```python
from build123d import *

# Parameters (mm, degrees)
ESQUISSE1_W              = 148
ESQUISSE1_H              = 330
BOSS_EXTRU_1_DEPTH       = 6
ESQUISSE2_W              = 30
ESQUISSE2_H              = 6
ESQUISSE2_W_2            = 6
ESQUISSE2_H_2            = 40
ENL_V_MAT_EXTRU_1_DEPTH  = 6
ESQUISSE6_W              = 6
ESQUISSE6_H              = 60
ENL_V_MAT_EXTRU_4_DEPTH  = 10
ESQUISSE8_W              = 6
ESQUISSE8_H              = 330
BOSS_EXTRU_2_DEPTH       = 57
ENL_V_MAT_EXTRU_5_DEPTH  = 389.536999525
ESQUISSE10_W             = 30
ESQUISSE10_H             = 6
ENL_V_MAT_EXTRU_6_DEPTH  = 389.536999525
ENL_V_MAT_EXTRU_9_DEPTH  = 389.536999525
ENL_V_MAT_EXTRU_11_DEPTH = 10
ESQUISSE16_R             = 1.5
ENL_V_MAT_EXTRU_12_DEPTH = 6
ESQUISSE17_R             = 2.995
ENL_V_MAT_EXTRU_13_DEPTH = 3
ESQUISSE18_R             = 9
ESQUISSE18_W             = 28.5
ESQUISSE18_H             = 12.5
ENL_V_MAT_EXTRU_14_DEPTH = 389.536999525
ESQUISSE5_W              = 30
ESQUISSE5_H              = 6
ESQUISSE5_H_2            = 3
ENL_V_MAT_EXTRU_15_DEPTH = 389.536999525


with BuildPart() as part:
    # Esquisse1 → Boss.-Extru.1 (new body)
    with BuildSketch(Plane.XY):
        with Locations((74, 165)):
            Rectangle(ESQUISSE1_W, ESQUISSE1_H)
    extrude(amount=BOSS_EXTRU_1_DEPTH)

    # Esquisse2 → Enlèv. mat.-Extru.1 (cut)
    with BuildSketch(Plane.XY.offset(6)):
        with Locations((45, 3)):
            Rectangle(ESQUISSE2_W, ESQUISSE2_H)
        with Locations((125, 3)):
            Rectangle(ESQUISSE2_W, ESQUISSE2_H)
        with Locations((45, 327)):
            Rectangle(ESQUISSE2_W, ESQUISSE2_H)
        with Locations((117, 327)):
            Rectangle(ESQUISSE2_W, ESQUISSE2_H)
        with Locations((3, 245)):
            Rectangle(ESQUISSE2_W_2, ESQUISSE2_H_2)
        with Locations((3, 165)):
            Rectangle(ESQUISSE2_W_2, ESQUISSE2_H_2)
        with Locations((3, 85)):
            Rectangle(ESQUISSE2_W_2, ESQUISSE2_H_2)
    extrude(amount=-ENL_V_MAT_EXTRU_1_DEPTH, mode=Mode.SUBTRACT)

    # Esquisse6 → Enlèv. mat.-Extru.4 (cut)
    with BuildSketch(Plane.XY.offset(6)):
        with Locations((107, 86)):
            Rectangle(ESQUISSE6_W, ESQUISSE6_H)
        with Locations((107, 194)):
            Rectangle(ESQUISSE6_W, ESQUISSE6_H)
    extrude(amount=-ENL_V_MAT_EXTRU_4_DEPTH, mode=Mode.SUBTRACT)

    # Esquisse8 → Boss.-Extru.2 (add)
    with BuildSketch(Plane(origin=(148, 0, 0), x_dir=(0, 0, -1), z_dir=(1, 0, 0))):
        with Locations((-3, 165)):
            Rectangle(ESQUISSE8_W, ESQUISSE8_H)
    extrude(amount=BOSS_EXTRU_2_DEPTH)

    # Esquisse9 → Enlèv. mat.-Extru.5 (cut, through all)
    with BuildSketch(Plane.XY.offset(6)):
        Polygon((165, 0), (205, 0), (205, 49), (165, 6), align=None)
        Polygon((165, 330), (205, 330), (205, 281), (165, 324), align=None)
    extrude(amount=-ENL_V_MAT_EXTRU_5_DEPTH, mode=Mode.SUBTRACT)

    # Esquisse10 → Enlèv. mat.-Extru.6 (cut, through all)
    with BuildSketch(Plane.XY.offset(6)):
        with Locations((135, 208)):
            Rectangle(ESQUISSE10_W, ESQUISSE10_H)
        with Locations((135, 122)):
            Rectangle(ESQUISSE10_W, ESQUISSE10_H)
    extrude(amount=-ENL_V_MAT_EXTRU_6_DEPTH, mode=Mode.SUBTRACT)

    # Esquisse13 → Enlèv. mat.-Extru.9 (cut, through all)
    with BuildSketch(Plane(origin=(0, 0, 0), x_dir=(-1, 0, 0), z_dir=(0, 0, -1))):
        Polygon((-88, 330), (-144, 330), (-144, 274), (-110, 274), (-110, 280), (-88, 280), align=None)
    extrude(amount=-ENL_V_MAT_EXTRU_9_DEPTH, mode=Mode.SUBTRACT)

    # Esquisse15 → Enlèv. mat.-Extru.11 (cut)
    with BuildSketch(Plane(origin=(0, 0, 0), x_dir=(-1, 0, 0), z_dir=(0, 0, -1))):
        Polygon((-110, 0), (-110, 116), (-104, 116), (-104, 164), (-110, 164), (-110, 280), (-88, 280), (-88, 330), (0, 330), (0, 0), align=None)
    extrude(amount=-ENL_V_MAT_EXTRU_11_DEPTH, mode=Mode.SUBTRACT)

    # Esquisse16 → Enlèv. mat.-Extru.12 (cut)
    with BuildSketch(Plane(origin=(0, 0, 0), x_dir=(-1, 0, 0), z_dir=(0, 0, -1))):
        with Locations((-152.5, 3)):
            Circle(ESQUISSE16_R)
        with Locations((-107, 123)):
            Circle(ESQUISSE16_R)
        with Locations((-107, 157)):
            Circle(ESQUISSE16_R)
        with Locations((-154.5, 327)):
            Circle(ESQUISSE16_R)
        with Locations((-157, 122)):
            Circle(ESQUISSE16_R)
        with Locations((-157, 208)):
            Circle(ESQUISSE16_R)
        with Locations((-113, 122)):
            Circle(ESQUISSE16_R)
        with Locations((-113, 208)):
            Circle(ESQUISSE16_R)
    extrude(amount=-ENL_V_MAT_EXTRU_12_DEPTH, mode=Mode.SUBTRACT)

    # Esquisse17 → Enlèv. mat.-Extru.13 (cut)
    with BuildSketch(Plane(origin=(0, 0, 0), x_dir=(-1, 0, 0), z_dir=(0, 0, -1))):
        with Locations((-152.5, 3)):
            Circle(ESQUISSE17_R)
        with Locations((-107, 123)):
            Circle(ESQUISSE17_R)
        with Locations((-107, 157)):
            Circle(ESQUISSE17_R)
        with Locations((-154.5, 327)):
            Circle(ESQUISSE17_R)
    extrude(amount=-ENL_V_MAT_EXTRU_13_DEPTH, mode=Mode.SUBTRACT)

    # Esquisse18 → Enlèv. mat.-Extru.14 (cut, through all)
    with BuildSketch(Plane(origin=(0, 0, 0), x_dir=(-1, 0, 0), z_dir=(0, 0, -1))):
        with Locations((-155, 25)):
            Circle(ESQUISSE18_R)
        with Locations((-159.25, 47.25)):
            Rectangle(ESQUISSE18_W, ESQUISSE18_H)
    extrude(amount=-ENL_V_MAT_EXTRU_14_DEPTH, mode=Mode.SUBTRACT)

    # Esquisse5 → Enlèv. mat.-Extru.15 (cut, through all)
    with BuildSketch(Plane.XY.offset(6)):
        with Locations((56.5, 277)):
            Rectangle(ESQUISSE5_W, ESQUISSE5_H)
        with Locations((56.5, 133.5)):
            Rectangle(ESQUISSE5_W, ESQUISSE5_H_2)
    extrude(amount=-ENL_V_MAT_EXTRU_15_DEPTH, mode=Mode.SUBTRACT)


solid = part.part
```
Verification items for the finished model (mm, model axes). A direction names the side the tool comes from. Give positions to 0.01 mm unless a question says otherwise; leave off trailing zeros. Order: outer loops, then holes, each group sorted by start corner. A loop starts at its lowest first (then second) coordinate and runs counter-clockwise, first axis right, second up. Notation, with made-up numbers: M 26.25,78 L 32.25,78 A21 ccw 32.25,105 Z; hole C 51.25,8.25 d4. An arc over 180 degrees is marked long. Return JSON: item names as keys, results as strings. Group by question number.
1) Scan lines: line 1 (Y direction, x = 113, z = 4.5); line 2 (Y direction, x = 138, z = 2.8); line 3 (Y direction, x = 158, z = 0.8). Record each from-to range of solid material in increasing order.
2) Go/stop test with flat-tipped pins: pin 1 Ø3 at (y, z) = (76.5, 3) entering from -X; pin 2 Ø3 at (x, z) = (135.5, 2) entering from -Y; pin 3 Ø2 at (x, z) = (132.5, 2) entering from +Y; pin 4 Ø1.8 at (x, y) = (107, 157) entering from -Z. Record where each tip stops, or that it passes through.
3) Mould release check, pull along X, two halves, no side actions. Record for faces 5 (the face through (185.28, 27.8, 3.04)), 6 (the face through (152, 0, 4)), 7 (the face through (152.89, 329.525, 1.479)): pulls with the +X half, pulls with the -X half, needs draft (parallel to the pull), parting line crosses it, or undercut.
4) Access from +Z, -Z, +X, -X, +Y, -Y to the whole of each face (thin tool, end or side, straight path). Record for faces 1 (the face through (120, 122, 3)), 2 (the face through (144, 302, 3)), 3 (the face through (140, 3, 3)), 4 (the face through (105.7, 121.7, 3)).
5) Section check C-C on y = 277.5. Record the cut outline in (x, z), and give its area (3 significant figures).
6) Section check A-A on y = 25. Record the cut outline in (x, z), and give its area (3 significant figures).
7) Section check D-D on x = 181. Record the cut outline in (y, z), and give its area (3 significant figures).
8) Section check B-B on z = 1.3. Give the number of separate pieces and of enclosed holes in the cut face, and give its area (3 significant figures).
Answer block:
{
 "1": {"line 1": "y = 6 to 120.5, 123.5 to 206.5, 209.5 to 274", "line 2": "y = 6 to 119, 125 to 205, 211 to 274", "line 3": "y = 0 to 16.51, 33.49 to 41, 53.5 to 120.88, 123.12 to 206.88, 209.12 to 330"},
 "2": {"pin 1": "stops at x = 110", "pin 2": "stops at y = 6", "pin 3": "stops at y = 274", "pin 4": "passes through"},
 "3": {"face 5": "pulls with the +X half", "face 6": "needs draft", "face 7": "undercut"},
 "4": {"face 1": "+Z, -Z", "face 2": "+Z, -Z, -X, +Y", "face 3": "+Z, -Z, -X, -Y", "face 4": "-Z"},
 "5": {"outline": "M 144,0 L 205,0 L 205,6 L 144,6 Z", "area": "366 mm^2"},
 "6": {"outline": "M 110,0 L 146,0 L 146,6 L 110,6 Z; M 164,0 L 182.67,0 L 182.67,6 L 164,6 Z", "area": "328 mm^2"},
 "7": {"outline": "M 23.2,0 L 306.8,0 L 306.8,6 L 23.2,6 Z", "area": "1,700 mm^2"},
 "8": {"separate pieces": "1", "enclosed holes": "12", "area": "26,200 mm^2"}
}
